Geometry: final body of the model. Coordinates: model frame, mm. Coordinates: 2 decimals unless noted, no trailing zeros. Order: outer loops, then holes, each group sorted by start corner. A loop starts at its lowest first (then second) coordinate and runs counter-clockwise, first axis right, second up. Notation, with made-up numbers: M 75.5,-22.5 L 100.5,-22.5 A23 ccw 100.5,2.5 Z; hole C 75,-25 d11. An arc over 180 degrees is marked long. Use CSV: the item, a comma, the result in double quotes. Start each with the question number.
1. First-contact query: P1, Ø2.5, axis at x = 0, z = 5, coming from the +Y side; P2, Ø2, axis at x = 9.5, y = -3.5, coming from the -Z side; P3, Ø5, axis at x = 3, z = 5.5, coming from the +Y side; P4, Ø3, axis at x = 4, z = 8.5, coming from the +Y side. Flat tips, straight axial feed; report the tip coordinate or a pass-through.
2. Material intervals for line 1 (Z direction, x = 0, y = 10); line 2 (X direction, y = 5.25, z = 8.5); line 3 (X direction, y = -10, z = 5), sorted ascending.
3. Section query B-B on x = 0. Return the cut outline in (y, z).
4. Section query C-C on z = 5. Return the cut outline in (x, y), and give its area (3 significant figures).
5. Section query A-A on y = 0. Return the cut outline in (x, z), and give its area (3 significant figures).
6. Section query D-D on z = 9. Return the cut outline in (x, y).
7. Pull-direction query (X, two-part tool) for faces 1 (the flat face through (-3, -5.4, 15)), 2 (the cylindrical face through (-0.195, -9.108, 3.513)), 3 (the cylindrical face through (11.923, -3.755, 7.395)); classes: pulls with the +X half, pulls with the -X half, needs draft (parallel to the pull), parting line crosses it, or undercut.
Autodesk Fusion 360 part; units mm, degrees
sketch "Sketch1" plane through (0, 0, 0) normal (0, 0, 1) x (1, 0, 0)
  circle A0 centre (0, 0) radius 12.5
  circle A1 centre (0, 0) radius 6
  dimension "d1" = 25
  dimension "d2" = 12
extrude "Extrude1" add sketch "Sketch1" along normal blind 15
sketch "Sketch2" plane through (0, 0, 0) normal (0, 1, 0) x (1, 0, 0)
  circle A0 centre (0, -5) radius 1.5
  dimension "d5" = 3
extrude "Extrude2" cut sketch "Sketch2" against normal blind 60
sketch "Sketch3" plane through (0, 0, 0) normal (0, 1, 0) x (-1, 0, 0)
  circle A0 centre (0, 5) radius 1.5
  dimension "d8" = 3
extrude "Extrude3" cut sketch "Sketch3" along normal blind 30
sketch "Sketch4" plane through (0, 0, 0) normal (0, 1, 0) x (1, 0, 0)
  circle A0 centre (0, -5) radius 1.5
  dimension "d9" = 3
Results list:
1,P1,"passes through"
1,P2,"stops at z = 0"
1,P3,"stops at y = 12.48"
1,P4,"stops at y = 12.25"
2,line 1,"z = 0 to 3.5, 6.5 to 15"
2,line 2,"x = -11.34 to -2.9, 2.9 to 11.34"
2,line 3,"x = -7.5 to -1.5, 1.5 to 7.5"
3,outline,"M -12.5,0 L -6,0 L -6,3.5 L -12.5,3.5 Z; M -12.5,6.5 L -6,6.5 L -6,15 L -12.5,15 Z; M 6,0 L 12.5,0 L 12.5,3.5 L 6,3.5 Z; M 6,6.5 L 12.5,6.5 L 12.5,15 L 6,15 Z"
4,outline,"M -1.5,-12.41 L -1.5,-5.81 A6 cw -1.5,5.81 L -1.5,12.41 A12.5 ccw Z; M 1.5,-12.41 A12.5 ccw 1.5,12.41 L 1.5,5.81 A6 cw 1.5,-5.81 Z"
4,area,"339 mm²"
5,outline,"M -12.5,0 L -6,0 L -6,15 L -12.5,15 Z; M 6,0 L 12.5,0 L 12.5,15 L 6,15 Z"
5,area,"195 mm²"
6,outline,"C 0,0 d25; hole C 0,0 d12"
7,face 1,"needs draft"
7,face 2,"undercut"
7,face 3,"parting line crosses it"
